Here's how the part is built. I have some questions about the finished solid (model axes, mm). Face numbers are marked on the shaded views. A direction names the side the tool comes from. Round coordinates to 2 decimals unless told otherwise and drop trailing zeros. Use a Markdown table: item, result.
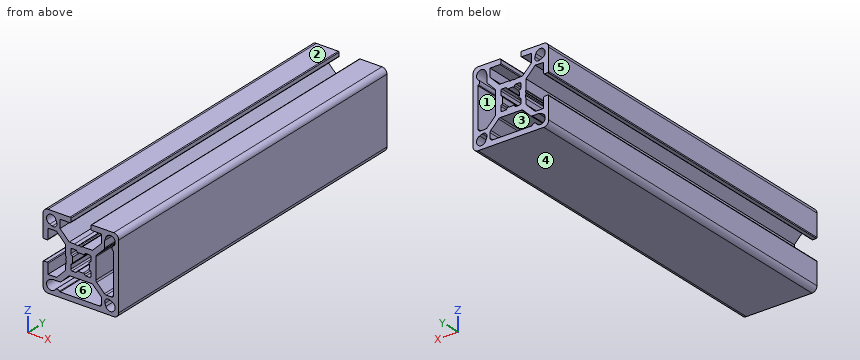
from build123d import *

# Parameters (mm, degrees)
F2_DEPTH = 70


# Not quite as in the source:
# - ends of sketch curves that miss each other by under 0.0002 mm in the source are joined


with BuildPart() as f2:
    # F1 (on Front) → F2 (new body, symmetric)
    with BuildSketch(Plane.XZ):
        with BuildLine():
            Line((-48.090856, 20.246586), (-44.140856, 20.246586))
            ThreePointArc((-44.140856, 20.246586), (-43.9287239656, 20.3344539656), (-43.840856, 20.546586))
            Line((-43.840856, 20.546586), (-43.840856, 21.946586))
            ThreePointArc((-43.840856, 21.946586), (-43.9287239656, 22.1587180344), (-44.140856, 22.246586))
            Line((-44.140856, 22.246586), (-52.840856, 22.246586))
            ThreePointArc((-52.840856, 22.246586), (-54.2550695624, 21.6607995624), (-54.840856, 20.246586))
            Line((-54.840856, 20.246586), (-54.840856, 11.546586))
            ThreePointArc((-54.840856, 11.546586), (-54.7529880344, 11.3344539656), (-54.540856, 11.246586))
            Line((-54.540856, 11.246586), (-53.140856, 11.246586))
            ThreePointArc((-53.140856, 11.246586), (-52.9287239656, 11.3344539656), (-52.840856, 11.546586))
            Line((-52.840856, 11.546586), (-52.840856, 15.496586))
            Line((-52.840856, 15.496586), (-49.50507, 15.496586))
            Line((-49.50507, 15.496586), (-45.840856, 11.832372))
            Line((-45.840856, 11.832372), (-45.840856, 7.900176))
            ThreePointArc((-45.840856, 7.900176), (-45.8238189324, 7.7707665494), (-45.7738687764, 7.6501761291))
            Line((-45.7738687764, 7.6501761291), (-45.540856, 7.246586))
            Line((-45.540856, 7.246586), (-45.773869, 6.842996))
            ThreePointArc((-45.773869, 6.842996), (-45.840856, 6.592996), (-45.7738687764, 6.3429961291))
            Line((-45.7738687764, 6.3429961291), (-45.591833, 6.0277))
            Line((-45.591833, 6.0277), (-45.840856, 4.746586))
            Line((-45.840856, 4.746586), (-45.840856, 2.6608))
            Line((-45.840856, 2.6608), (-49.50507, -1.003414))
            Line((-49.50507, -1.003414), (-52.840856, -1.003414))
            Line((-52.840856, -1.003414), (-52.840856, 2.946586))
            ThreePointArc((-52.840856, 2.946586), (-52.9287239656, 3.1587180344), (-53.140856, 3.246586))
            Line((-53.140856, 3.246586), (-54.540856, 3.246586))
            ThreePointArc((-54.540856, 3.246586), (-54.7529880344, 3.1587180344), (-54.840856, 2.946586))
            Line((-54.840856, 2.946586), (-54.840856, -5.753414))
            ThreePointArc((-54.840856, -5.753414), (-54.2550695624, -7.1676275624), (-52.840856, -7.753414))
            Line((-52.840856, -7.753414), (-26.840856, -7.753414))
            ThreePointArc((-26.840856, -7.753414), (-25.4266424376, -7.1676275624), (-24.840856, -5.753414))
            Line((-24.840856, -5.753414), (-24.840856, 20.246586))
            ThreePointArc((-24.840856, 20.246586), (-25.4266424376, 21.6607995624), (-26.840856, 22.246586))
            Line((-26.840856, 22.246586), (-35.540856, 22.246586))
            ThreePointArc((-35.540856, 22.246586), (-35.7529880344, 22.1587180344), (-35.840856, 21.946586))
            Line((-35.840856, 21.946586), (-35.840856, 20.546586))
            ThreePointArc((-35.840856, 20.546586), (-35.7529880344, 20.3344539656), (-35.540856, 20.246586))
            Line((-35.540856, 20.246586), (-31.590856, 20.246586))
            Line((-31.590856, 20.246586), (-31.590856, 16.9108))
            Line((-31.590856, 16.9108), (-35.25507, 13.246586))
            Line((-35.25507, 13.246586), (-39.187266, 13.246586))
            ThreePointArc((-39.187266, 13.246586), (-39.3166754506, 13.2295489324), (-39.4372658709, 13.1795987764))
            Line((-39.4372658709, 13.1795987764), (-39.840856, 12.946586))
            Line((-39.840856, 12.946586), (-40.244446, 13.179599))
            ThreePointArc((-40.244446, 13.179599), (-40.494446, 13.246586), (-40.7444458709, 13.1795987764))
            Line((-40.7444458709, 13.1795987764), (-41.059742, 12.997563))
            Line((-41.059742, 12.997563), (-42.340856, 13.246586))
            Line((-42.340856, 13.246586), (-44.426642, 13.246586))
            Line((-44.426642, 13.246586), (-48.090856, 16.9108))
            Line((-48.090856, 16.9108), (-48.090856, 20.246586))
        make_face()
        with BuildLine():
            ThreePointArc((-48.030175, -5.753414), (-48.180175082, -5.7132215738), (-48.2899827159, -5.6034138359))
            ThreePointArc((-48.2899827159, -5.6034138359), (-49.1151948384, -5.1042472042), (-49.9783690315, -5.5344479782))
            ThreePointArc((-49.9783690315, -5.5344479782), (-53.0449723505, -5.6142903949), (-52.1906940253, -2.6679979306))
            Line((-52.1906940253, -2.6679979306), (-50.91426, -2.203414))
            Line((-50.91426, -2.203414), (-48.290856, -2.203414))
            ThreePointArc((-48.290856, -2.203414), (-47.9081725676, -2.1272935325), (-47.5837492188, -1.9105207812))
            Line((-47.5837492188, -1.9105207812), (-44.719536, 0.953693))
            ThreePointArc((-44.719536, 0.953693), (-44.3951124324, 1.1704655325), (-44.012429, 1.246586))
            Line((-44.012429, 1.246586), (-35.669283, 1.246586))
            ThreePointArc((-35.669283, 1.246586), (-35.2865995676, 1.1704655325), (-34.9621762188, 0.9536927812))
            Line((-34.9621762188, 0.9536927812), (-31.883749, -2.124734))
            ThreePointArc((-31.883749, -2.124734), (-31.6669764675, -2.4491575676), (-31.590856, -2.831841))
            Line((-31.590856, -2.831841), (-31.590856, -4.753414))
            ThreePointArc((-31.590856, -4.753414), (-31.8837492188, -5.4605207812), (-32.590856, -5.753414))
            Line((-32.590856, -5.753414), (-48.030175, -5.753414))
        make_face(mode=Mode.SUBTRACT)
        with BuildLine():
            ThreePointArc((-30.2930043339, -4.0956641215), (-29.9673844937, -2.6268855063), (-28.4986058785, -2.3012656661))
            Line((-28.4986058785, -2.3012656661), (-27.491018, -2.667998))
            ThreePointArc((-27.491018, -2.667998), (-26.7973531157, -5.7969168843), (-29.9262720694, -5.1032520253))
            Line((-29.9262720694, -5.1032520253), (-30.2930043339, -4.0956641215))
        make_face(mode=Mode.SUBTRACT)
        with BuildLine():
            ThreePointArc((-36.5876690145, 8.2349049956), (-36.440856, 7.246586), (-36.5876690145, 6.2582670044))
            ThreePointArc((-36.5876690145, 6.2582670044), (-36.5433888407, 5.9288023569), (-36.2653470651, 5.7465855742))
            ThreePointArc((-36.2653470651, 5.7465855742), (-35.9615444769, 5.5780848975), (-35.840856, 5.25232))
            Line((-35.840856, 5.25232), (-35.840856, 3.746586))
            ThreePointArc((-35.840856, 3.746586), (-35.9873026094, 3.3930326094), (-36.340856, 3.246586))
            Line((-36.340856, 3.246586), (-37.84659, 3.246586))
            ThreePointArc((-37.84659, 3.246586), (-38.1723548975, 3.3672744769), (-38.3408555178, 3.6710770737))
            ThreePointArc((-38.3408555178, 3.6710770737), (-38.5230723569, 3.9491188407), (-38.8525409519, 3.9933978415))
            ThreePointArc((-38.8525409519, 3.9933978415), (-39.840856, 3.846586), (-40.8291749956, 3.9933990145))
            ThreePointArc((-40.8291749956, 3.9933990145), (-41.1586396431, 3.9491188407), (-41.3408564258, 3.6710770651))
            ThreePointArc((-41.3408564258, 3.6710770651), (-41.5093571025, 3.3672744769), (-41.835122, 3.246586))
            Line((-41.835122, 3.246586), (-43.340856, 3.246586))
            ThreePointArc((-43.340856, 3.246586), (-43.6944093906, 3.3930326094), (-43.840856, 3.746586))
            Line((-43.840856, 3.746586), (-43.840856, 5.25232))
            ThreePointArc((-43.840856, 5.25232), (-43.7201675231, 5.5780848975), (-43.4163649263, 5.7465855178))
            ThreePointArc((-43.4163649263, 5.7465855178), (-43.1383231593, 5.9288023569), (-43.0940441585, 6.2582709519))
            ThreePointArc((-43.0940441585, 6.2582709519), (-43.240856, 7.246586), (-43.0940429855, 8.2349049956))
            ThreePointArc((-43.0940429855, 8.2349049956), (-43.1383231593, 8.5643696431), (-43.4163649349, 8.7465864258))
            ThreePointArc((-43.4163649349, 8.7465864258), (-43.7201675231, 8.9150871025), (-43.840856, 9.240852))
            Line((-43.840856, 9.240852), (-43.840856, 10.746586))
            ThreePointArc((-43.840856, 10.746586), (-43.6944093906, 11.1001393906), (-43.340856, 11.246586))
            Line((-43.340856, 11.246586), (-41.835122, 11.246586))
            ThreePointArc((-41.835122, 11.246586), (-41.5093571025, 11.1258975231), (-41.3408564822, 10.8220949263))
            ThreePointArc((-41.3408564822, 10.8220949263), (-41.1586396431, 10.5440531593), (-40.8291710481, 10.4997741585))
            ThreePointArc((-40.8291710481, 10.4997741585), (-39.840856, 10.646586), (-38.8525370044, 10.4997729855))
            ThreePointArc((-38.8525370044, 10.4997729855), (-38.5230723569, 10.5440531593), (-38.3408555742, 10.8220949349))
            ThreePointArc((-38.3408555742, 10.8220949349), (-38.1723548975, 11.1258975231), (-37.84659, 11.246586))
            Line((-37.84659, 11.246586), (-36.340856, 11.246586))
            ThreePointArc((-36.340856, 11.246586), (-35.9873026094, 11.1001393906), (-35.840856, 10.746586))
            Line((-35.840856, 10.746586), (-35.840856, 9.240852))
            ThreePointArc((-35.840856, 9.240852), (-35.9615444769, 8.9150871025), (-36.2653470737, 8.7465864822))
            ThreePointArc((-36.2653470737, 8.7465864822), (-36.5433888407, 8.5643696431), (-36.5876690145, 8.2349049956))
        make_face(mode=Mode.SUBTRACT)
        with BuildLine():
            ThreePointArc((-49.3887076661, 18.5888361215), (-49.7143275063, 17.1200575063), (-51.1831061215, 16.7944376661))
            Line((-51.1831061215, 16.7944376661), (-52.190694, 17.16117))
            ThreePointArc((-52.190694, 17.16117), (-52.8843588843, 20.2900888843), (-49.7554399306, 19.5964240253))
            Line((-49.7554399306, 19.5964240253), (-49.3887076661, 18.5888361215))
        make_face(mode=Mode.SUBTRACT)
        with BuildLine():
            ThreePointArc((-33.5479627812, 2.3679062188), (-33.7647355325, 2.6923295676), (-33.840856, 3.075013))
            Line((-33.840856, 3.075013), (-33.840856, 11.418159))
            ThreePointArc((-33.840856, 11.418159), (-33.7647355325, 11.8008424324), (-33.5479627812, 12.1252657812))
            Line((-33.5479627812, 12.1252657812), (-30.683749, 14.989479))
            ThreePointArc((-30.683749, 14.989479), (-30.4669764675, 15.3139025676), (-30.390856, 15.696586))
            Line((-30.390856, 15.696586), (-30.390856, 18.31999))
            Line((-30.390856, 18.31999), (-29.926272, 19.596424))
            ThreePointArc((-29.926272, 19.596424), (-26.9799796051, 20.4507023505), (-27.0598220201, 17.3840990291))
            ThreePointArc((-27.0598220201, 17.3840990291), (-27.4900227958, 16.5209248384), (-26.9908561748, 15.6957126972))
            ThreePointArc((-26.9908561748, 15.6957126972), (-26.8810484262, 15.585905082), (-26.840856, 15.435905))
            Line((-26.840856, 15.435905), (-26.840856, -0.003414))
            ThreePointArc((-26.840856, -0.003414), (-27.1337492188, -0.7105207812), (-27.840856, -1.003414))
            Line((-27.840856, -1.003414), (-29.762429, -1.003414))
            ThreePointArc((-29.762429, -1.003414), (-30.1451124324, -0.9272935325), (-30.4695357812, -0.7105207812))
            Line((-30.4695357812, -0.7105207812), (-33.5479627812, 2.3679062188))
        make_face(mode=Mode.SUBTRACT)
    extrude(amount=F2_DEPTH, both=True)


solid = f2.part
1. We'd pull the mould along Z, two halves only. Please class the marked faces 3, 4, 5 and 6: +Z half, -Z half, draft (parallel to the pull), parting line (faces both ways), or undercut.
Answer sheet:
| item | result |
|---|---|
| face 3 | undercut |
| face 4 | -Z half |
| face 5 | draft |
| face 6 | undercut |
2. I need wall thicknesses on probe 1 along X at (y, z) = (-18, 11.5); probe 2 along Z at (x, y) = (-37.5, 5); probe 3 along X at (y, z) = (29, 9.5). Which ranges of each line are inside material? Lowest first, please. Write a range as from..to.
Answer sheet:
| item | result |
|---|---|
| probe 1 | -54.84..-52.84, -45.84..-33.84, -26.84..-24.84 |
| probe 2 | -7.75..-5.75, 1.25..3.25, 11.25..13.25 |
| probe 3 | -45.84..-43.84, -35.84..-33.84, -26.84..-24.84 |
3. Imagine slicing it at A-A, the plane y = 57. State how many separate pieces and enclosed holes the cut face has, then the cut area to 3 significant figures.
Answer sheet:
| item | result |
|---|---|
| separate pieces | 1 |
| enclosed holes | 5 |
| area | 339 mm2 |
4. For pin 1 Ø10 at (x, y) = (-37, -35) entering from +Z; pin 2 Ø1.2 at (y, z) = (3, 9) entering from -X; pin 3 Ø0.7 at (y, z) = (6.5, 21.5) entering from +X; pin 4 Ø2.5 at (x, z) = (-51.54, 18.95) entering from +Y, each with a flat end and sliding along its axis, tell me the tip position at first contact or that it passes through.
Answer sheet:
| item | result |
|---|---|
| pin 1 | z = 22.25 |
| pin 2 | x = -45.84 |
| pin 3 | x = -25.06 |
| pin 4 | through |
5. Which directions (+Z, -Z, +X, -X, +Y, -Y) give clear straight access to the entire face, cutting with the end or side of a thin tool? Please do the marked faces 1 and 2.
Answer sheet:
| item | result |
|---|---|
| face 1 | +Y, -Y |
| face 2 | +Z, +X, -X, +Y, -Y |
